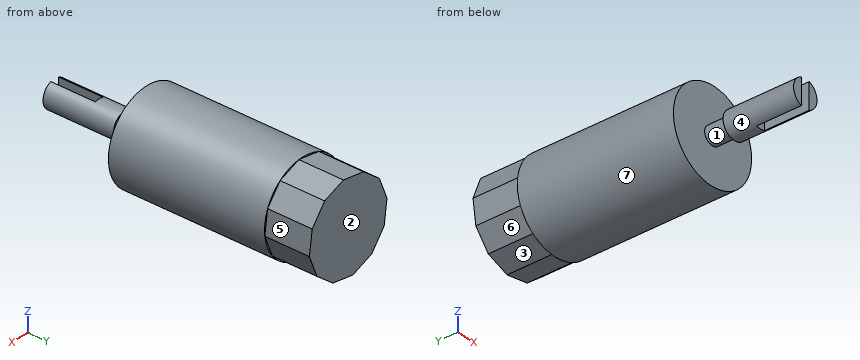
```python
from build123d import *

# Parameters (mm, degrees)
SKETCH_1_R          = 1.5
EXTRUDE_1_DEPTH     = 7.9
CUT_EXTRUDE_1_DEPTH = 5
SKETCH_3_R          = 1
EXTRUDE_2_DEPTH     = 2.5
SKETCH_4_R          = 5
EXTRUDE_3_DEPTH     = 22.5
CUT_EXTRUDE_START   = -5
CUT_EXTRUDE_3_DEPTH = 5


with BuildPart() as part:
    # 草图1 → 凸台-拉伸1 (new body)
    with BuildSketch(Plane(origin=(0, 0, 0), x_dir=(1, 0, 0), z_dir=(0, 1, 0))):
        with Locations(Location((0, 0, 0), (0, 0, 270))):
            Circle(SKETCH_1_R)
    extrude(amount=EXTRUDE_1_DEPTH)

    # 草图2 → 切除-拉伸1 (cut)
    with BuildSketch(Plane.XZ):
        with BuildLine():
            Line((-0.5, 1.414213562), (-0.5, -1.414213562))
            ThreePointArc((-0.5, -1.414213562), (0, -1.5), (0.5, -1.414213562))
            Line((0.5, -1.414213562), (0.5, 1.414213562))
            ThreePointArc((0.5, 1.414213562), (0, 1.5), (-0.5, 1.414213562))
        make_face()
    extrude(amount=-CUT_EXTRUDE_1_DEPTH, mode=Mode.SUBTRACT)

    # 草图3 → 凸台-拉伸2 (add)
    with BuildSketch(Plane(origin=(0, 7.9, 0), x_dir=(1, 0, 0), z_dir=(0, 1, 0))):
        with Locations(Location((0, 0, 0), (0, 0, 270))):
            Circle(SKETCH_3_R)
    extrude(amount=EXTRUDE_2_DEPTH)

    # 草图4 → 凸台-拉伸3 (add)
    with BuildSketch(Plane(origin=(0, 10.4, 0), x_dir=(1, 0, 0), z_dir=(0, 1, 0))):
        with Locations(Location((0, 0, 0), (0, 0, 90))):
            Circle(SKETCH_4_R)
    extrude(amount=EXTRUDE_3_DEPTH)

    # 草图5 → 切除-拉伸3 (cut)
    with BuildSketch(Plane(origin=(0, 32.9, 0), x_dir=(1, 0, 0), z_dir=(0, 1, 0)).offset(CUT_EXTRUDE_START)):
        with BuildLine():
            ThreePointArc((-1.954985899, -4.60195938), (-0.697296637, -4.951139), (0.607912238, -4.96290668))
            Line((0.607912238, -4.96290668), (-1.954985899, -4.60195938))
        make_face()
        with BuildLine():
            ThreePointArc((0.607912238, -4.96290668), (1.871692898, -4.63646047), (3.007920781, -3.994047142))
            Line((3.007920781, -3.994047142), (0.607912238, -4.96290668))
        make_face()
        with BuildLine():
            ThreePointArc((3.007920781, -3.994047142), (3.939163833, -3.079446102), (4.60195938, -1.954985899))
            Line((4.60195938, -1.954985899), (3.007920781, -3.994047142))
        make_face()
        with BuildLine():
            ThreePointArc((5, 0), (4.990718054, 0.304521429), (4.96290668, 0.607912238))
            Line((4.96290668, 0.607912238), (4.60195938, -1.954985899))
            ThreePointArc((4.60195938, -1.954985899), (4.899479406, -0.997547768), (5, 0))
        make_face()
        with BuildLine():
            ThreePointArc((4.96290668, 0.607912238), (4.63646047, 1.871692898), (3.994047142, 3.007920781))
            Line((3.994047142, 3.007920781), (4.96290668, 0.607912238))
        make_face()
        with BuildLine():
            Line((-1.954985899, -4.60195938), (-3.994047142, -3.007920781))
            ThreePointArc((-3.994047142, -3.007920781), (-3.079446102, -3.939163833), (-1.954985899, -4.60195938))
        make_face()
        with BuildLine():
            Line((-3.994047142, -3.007920781), (-4.96290668, -0.607912238))
            ThreePointArc((-4.96290668, -0.607912238), (-4.63646047, -1.871692898), (-3.994047142, -3.007920781))
        make_face()
        with BuildLine():
            Line((-4.96290668, -0.607912238), (-4.60195938, 1.954985899))
            ThreePointArc((-4.60195938, 1.954985899), (-4.951139, 0.697296637), (-4.96290668, -0.607912238))
        make_face()
        with BuildLine():
            Line((-4.60195938, 1.954985899), (-3.007920781, 3.994047142))
            ThreePointArc((-3.007920781, 3.994047142), (-3.939163833, 3.079446102), (-4.60195938, 1.954985899))
        make_face()
        with BuildLine():
            Line((-3.007920781, 3.994047142), (-0.607912238, 4.96290668))
            ThreePointArc((-0.607912238, 4.96290668), (-1.871692898, 4.63646047), (-3.007920781, 3.994047142))
        make_face()
        with BuildLine():
            Line((-0.607912238, 4.96290668), (1.954985899, 4.60195938))
            ThreePointArc((1.954985899, 4.60195938), (0.697296637, 4.951139), (-0.607912238, 4.96290668))
        make_face()
        with BuildLine():
            ThreePointArc((3.994047142, 3.007920781), (3.079446102, 3.939163833), (1.954985899, 4.60195938))
            Line((1.954985899, 4.60195938), (3.994047142, 3.007920781))
        make_face()
    extrude(amount=CUT_EXTRUDE_3_DEPTH, mode=Mode.SUBTRACT)


solid = part.part
```
Could you check a few things on this model? Use its own coordinates, in mm. Face numbers are marked on the shaded views. A direction names the side the tool comes from. Give positions to 0.01 mm unless a question says otherwise; leave off trailing zeros. Write each loop counter-clockwise with the first axis right and the second up, starting at its lowest first coordinate (ties: lowest second). Pieces come first, ordered by that corner, then holes. Notation, with made-up numbers: (86, 73.5) - (94, 73.5) arc R9 cw to (94, 77.5) - close; hole circle Ø5 at (51.5, 43.25). An arc over 180 degrees is marked (long way). One line per item, written item: value. Start each with the question number.
Item 1: Imagine slicing it at C-C, the plane x = 3.5. List the corners of the cut face in (y, z) for me, and give its area (3 significant figures).
Item 2: Which directions (+Z, -Z, +X, -X, +Y, -Y) give clear straight access to the entire face, cutting with the end or side of a thin tool? Please do the marked faces 4, 5, 6 and 7.
Item 3: If we mould it in two halves opening along Y, with no side actions, what happens to the marked faces 1, 2 and 3? For each: +Y half, -Y half, draft (parallel to the pull), parting line (faces both ways), or undercut.
Item 4: Please list where these lines run through material, in increasing order: line 1 (Y direction, x = 4.25, z = 2); line 2 (Y direction, x = 0, z = 0.5); line 3 (X direction, y = 19.5, z = -3). Write a range as from..to.
Item 5: Imagine slicing it at B-B, the plane z = 0. List the corners of the cut face in (x, y) for me.
Item 6: Imagine slicing it at A-A, the plane y = 28.5. List the corners of the cut face in (x, z) for me, and give its area (3 significant figures).
Item 7: I'm going to push flat-ended pins straight in: pin 1 (4 mm diameter, centred on y = 5, z = 1.5, fed in from -X); pin 2 (1.4 mm diameter, centred on y = 2.5, z = -0.5, fed in from +X). Where does each tip first touch, or does it pass through?
Item 8: Imagine slicing it at D-D, the plane y = 10. List the corners of the cut face in (x, z) for me.
Geometry says:
1. outline: (10.4, -3.57) - (27.9, -3.57) - (27.9, -3.39) - (32.9, -3.39) - (32.9, 3.36) - (27.9, 3.36) - (27.9, 3.57) - (10.4, 3.57) - close
1. area: 159 mm^2
2. face 4: -Y
2. face 5: +Z, +X, +Y
2. face 6: -Z, -X, +Y
2. face 7: +Y, -Y
3. face 1: undercut
3. face 2: +Y half
3. face 3: draft
4. line 1: 10.4..32.9
4. line 2: 5..32.9
4. line 3: -4..4
5. outline: (-5, 10.4) - (-1, 10.4) - (-1, 7.9) - (-1.5, 7.9) - (-1.5, 0) - (-0.5, 0) - (-0.5, 5) - (0.5, 5) - (0.5, 0) - (1.5, 0) - (1.5, 7.9) - (1, 7.9) - (1, 10.4) - (5, 10.4) - (5, 27.9) - (4.88, 27.9) - (4.88, 32.9) - (-4.88, 32.9) - (-4.88, 27.9) - (-5, 27.9) - close
6. outline: (-4.96, 0.61) - (-4.6, -1.95) - (-3.01, -3.99) - (-0.61, -4.96) - (1.95, -4.6) - (3.99, -3.01) - (4.96, -0.61) - (4.6, 1.95) - (3.01, 3.99) - (0.61, 4.96) - (-1.95, 4.6) - (-3.99, 3.01) - close
6. area: 75.0 mm^2
7. pin 1: x = -1.5
7. pin 2: x = 1.5
8. outline: circle Ø2 at (0, 0)
